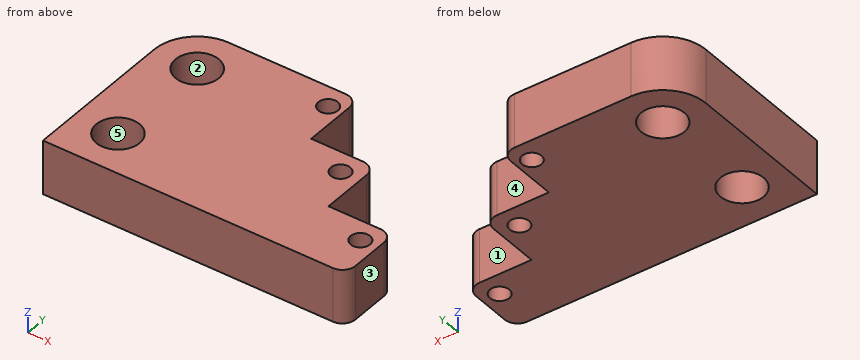
```python
from build123d import *

# Parameters (mm, degrees)
F0_R     = 10
F0_R_2   = 4.5
F1_DEPTH = 25


with BuildPart() as f1:
    # F0 (on Top) → F1 (new body)
    with BuildSketch(Plane.XY):
        with BuildLine():
            ThreePointArc((-65.204328, 54.130437), (-79.346463, 48.272573), (-85.204328, 34.130437))
            Line((-85.204328, 34.130437), (-85.204328, -15.869563))
            ThreePointArc((-85.204328, -15.869563), (-79.346463, -30.011699), (-65.204328, -35.869563))
            Line((-65.204328, -35.869563), (48.795672, -35.869563))
            ThreePointArc((48.795672, -35.869563), (53.038313, -34.112204), (54.795672, -29.869563))
            Line((54.795672, -29.869563), (54.795672, -11.869563))
            ThreePointArc((54.795672, -11.869563), (53.038313, -7.626922), (48.795672, -5.869563))
            Line((48.795672, -5.869563), (24.795672, -5.869563))
            Line((24.795672, -5.869563), (24.795672, 18.130437))
            ThreePointArc((24.795672, 18.130437), (23.038313, 22.373078), (18.795672, 24.130437))
            Line((18.795672, 24.130437), (-5.204328, 24.130437))
            Line((-5.204328, 24.130437), (-5.204328, 48.130437))
            ThreePointArc((-5.204328, 48.130437), (-6.961687, 52.373078), (-11.204328, 54.130437))
            Line((-11.204328, 54.130437), (-65.204328, 54.130437))
        make_face()
        with Locations((-65.204328, -15.869563)):
            Circle(F0_R, mode=Mode.SUBTRACT)
        with Locations((46.84058, -15.869563)):
            Circle(F0_R_2, mode=Mode.SUBTRACT)
        with Locations((-65.204328, 34.130437)):
            Circle(F0_R, mode=Mode.SUBTRACT)
        with Locations((15.724638, 14.130437)):
            Circle(F0_R_2, mode=Mode.SUBTRACT)
        with Locations((-12, 44.130437)):
            Circle(F0_R_2, mode=Mode.SUBTRACT)
        with BuildLine():
            ThreePointArc((-65.204328, -35.869563), (-79.346463, -30.011699), (-85.204328, -15.869563))
            Line((-85.204328, -15.869563), (-85.204328, -35.869563))
            Line((-85.204328, -35.869563), (-65.204328, -35.869563))
        make_face()
    extrude(amount=F1_DEPTH)


solid = f1.part
```
Geometry: final body of the model. Coordinates: model frame, mm. Face numbers are marked on the shaded views. A direction names the side the tool comes from. Round coordinates to 2 decimals unless told otherwise and drop trailing zeros. Loops run counter-clockwise (first coordinate to the right, second up) from the corner with the lowest first, then second, coordinate; pieces in that order, holes last. Notation, with made-up numbers: (-6.75, 25.25) -> (10.25, 25.25) arc R21 ccw to (10.25, 57.25) -> close; hole circle Ø4 at (66.25, 49). An arc over 180 degrees is marked (long way). Use one line per item in the form item = value. Start each with the question number.
1) Draft query along Y for the marked faces 3, 4 and 5. Return one class per face: released by +Y, released by -Y, zero draft, split by the parting line, or undercut.
2) Section D-D on x = 7. Output: boundary loops of the cut face in (y, z).
3) Section A-A on y = -23.5. Output: boundary loops of the cut face in (x, z).
4) Section C-C on x = 37.5. Output: boundary loops of the cut face in (y, z), then the cut area to 3 significant figures.
5) Access query for the marked faces 1 and 2. Directions: +Z, -Z, +X, -X, +Y, -Y. A direction counts if a zero-diameter tool reaches every point of the face in a straight line with its end or side. Return the directions, or none.
6) Line query: L1, parallel to X at y = 41.5, z = 14.75; L2, parallel to X at y = 11.5, z = 2.25; L3, parallel to X at y = 34, z = 4.25. Output: solid intervals per line, ascending.
7) Section B-B on z = 9.75. Output: boundary loops of the cut face in (x, y), then the cut area to 3 significant figures.
8) First-contact query: P1, Ø2, axis at y = 28.5, z = 4, coming from the +X side; P2, Ø12, axis at x = 10.5, z = 8.5, coming from the +Y side; P3, Ø5, axis at y = 42.5, z = 6, coming from the -X side. Flat tips, straight axial feed; report the tip coordinate or a pass-through.
Response:
q1.face_3 = zero draft
q1.face_4 = released by +Y
q1.face_5 = undercut
q2.outline = (-35.87, 0) -> (24.13, 0) -> (24.13, 25) -> (-35.87, 25) -> close
q3.outline = (-85.2, 0) -> (-71.67, 0) -> (-71.67, 25) -> (-85.2, 25) -> close; (-58.74, 0) -> (54.8, 0) -> (54.8, 25) -> (-58.74, 25) -> close
q4.outline = (-35.87, 0) -> (-5.87, 0) -> (-5.87, 25) -> (-35.87, 25) -> close
q4.area = 750 mm^2
q5.face_1 = +Z, -Z, +X, +Y
q5.face_2 = +Z, -Z
q6.L1 = -83.8 to -71.96, -58.44 to -15.65, -8.35 to -5.2
q6.L2 = -85.2 to 12.07, 19.38 to 24.8
q6.L3 = -85.2 to -75.2, -55.21 to -5.2
q7.outline = (-85.2, -35.87) -> (48.8, -35.87) arc R6 ccw to (54.8, -29.87) -> (54.8, -11.87) arc R6 ccw to (48.8, -5.87) -> (24.8, -5.87) -> (24.8, 18.13) arc R6 ccw to (18.8, 24.13) -> (-5.2, 24.13) -> (-5.2, 48.13) arc R6 ccw to (-11.2, 54.13) -> (-65.2, 54.13) arc R20 ccw to (-85.2, 34.13) -> close; hole circle Ø20 at (-65.2, -15.87); hole circle Ø20 at (-65.2, 34.13); hole circle Ø9 at (-12, 44.13); hole circle Ø9 at (15.72, 14.13); hole circle Ø9 at (46.84, -15.87)
q7.area = 8,960 mm^2
q8.P1 = -5.2
q8.P2 = 24.13
q8.P3 = -84.32
